Could you check a few things on this model? Use its own coordinates, in mm. Face numbers are marked on the shaded views. Give positions to 0.01 mm unless a question says otherwise; leave off trailing zeros. Order: outer loops, then holes, each group sorted by start corner. A loop starts at its lowest first (then second) coordinate and runs counter-clockwise, first axis right, second up. Notation, with made-up numbers: (69.25, -17) - (87.25, -17) arc R19 cw to (87.25, 8) - close; hole circle Ø4 at (13.25, 81). An arc over 180 degrees is marked (long way). One line per question, with ' | ' between items. Start each with the question number.
1. Imagine slicing it at D-D (x = 62). Please give me the cut outline in (y, z).
2. Imagine slicing it at C-C (z = -45.9). Please give me the cut outline in (x, y), and give its area (3 significant figures).
3. If we mould it in two halves opening along Z, with no side actions, what happens to the marked faces 1 and 2? For each: released by +Z, released by -Z, zero draft, split by the parting line, or undercut.
4. Imagine slicing it at A-A (z = -17.94). Please give me the cut outline in (x, y).
5. Imagine slicing it at B-B (y = 2.95). Give the number of separate pieces and of enclosed holes in the cut face, and give its area (3 significant figures).
6. I need wall thicknesses on probe 1 along Z at (x, y) = (1, 3.65); probe 2 along Y at (x, z) = (63.5, -30); probe 3 along X at (y, z) = (1.6, -8.5). Which ranges of each line are inside material? Lowest first, please. Write a range as from..to.
7. For P1, Ø3, axis at y = 3, z = -45, coming from the +X side; P2, Ø2, axis at x = 54.12, z = -50.9, coming from the -Y side; P3, Ø2, axis at x = 42.5, y = 4.5, coming from the +Z side; P4, Ø1, axis at x = 54.5, z = -51, coming from the +Y side, each with a flat end and sliding along its axis, tell me the tip position at first contact or that it passes through.
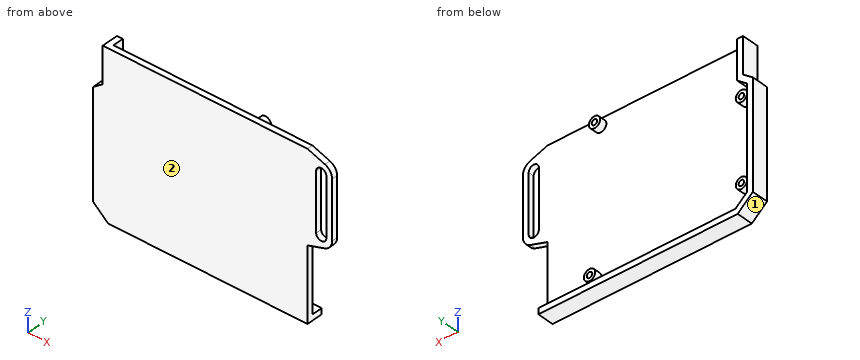
```python
from build123d import *

# Parameters (mm, degrees)
SALIENTE_EXTRUIR2_DEPTH = 2
SALIENTE_EXTRUIR3_DEPTH = 3.7
CROQUIS3_R              = 1.95
CROQUIS3_R_2            = 0.95
SALIENTE_EXTRUIR4_DEPTH = 2.5


with BuildPart() as part:
    # Croquis1 → Saliente-Extruir2 (new body)
    with BuildSketch(Plane(origin=(0, 0, 0), x_dir=(1, 0, 0), z_dir=(0, 1, 0))):
        with BuildLine():
            Line((70.799071053, 31.092568315), (70.799071053, 56.4))
            Line((70.799071053, 56.4), (1.865918726, 56.4))
            Line((1.865918726, 56.4), (-3.400928947, 51.75405083))
            Line((-3.400928947, 51.75405083), (-3.400928947, 14.921940047))
            Line((-3.400928947, 14.921940047), (0, 12.421940047))
            Line((0, 12.421940047), (0, 0))
            Line((0, 0), (70.799071053, 0))
            Line((70.799071053, 0), (76.842269578, 2.170786153))
            ThreePointArc((76.842269578, 2.170786153), (78.641822821, 3.542629227), (79.324535526, 5.7))
            Line((79.324535526, 5.7), (79.324535526, 25.7))
            ThreePointArc((79.324535526, 25.7), (78.590944159, 27.927953986), (76.677186746, 29.284223805))
            Line((76.677186746, 29.284223805), (70.799071053, 31.092568315))
        make_face()
        with BuildLine():
            Line((77.324535526, 25.7), (77.324535526, 5.7))
            ThreePointArc((77.324535526, 5.7), (75.574535526, 3.95), (73.824535526, 5.7))
            Line((73.824535526, 5.7), (73.824535526, 25.7))
            ThreePointArc((73.824535526, 25.7), (75.574535526, 27.45), (77.324535526, 25.7))
        make_face(mode=Mode.SUBTRACT)
    extrude(amount=SALIENTE_EXTRUIR2_DEPTH)

    # Croquis2 → Saliente-Extruir3 (add)
    with BuildSketch(Plane(origin=(0, 2, 0), x_dir=(1, 0, 0), z_dir=(0, 1, 0))):
        Polygon((70.799071053, 54.4), (2.621972909, 54.4), (-1.400928947, 50.851350277), (-1.400928947, 15.933980016), (2, 13.433980016), (2, 0), (0, 0), (0, 12.421940047), (-3.400928947, 14.921940047), (-3.400928947, 51.75405083), (1.865918726, 56.4), (70.799071053, 56.4), align=None)
    extrude(amount=SALIENTE_EXTRUIR3_DEPTH)

    # Croquis3 → Saliente-Extruir4 (add)
    # profile 1 of 4: a face of its own
    with BuildSketch(Plane(origin=(0, 2, 0), x_dir=(1, 0, 0), z_dir=(0, 1, 0))):
        with Locations(Location((1.599071053, 45.9, 0), (0, 0, 270))):
            Circle(CROQUIS3_R)
        with Locations(Location((1.599071053, 45.9, 0), (0, 0, 270))):
            Circle(CROQUIS3_R_2, mode=Mode.SUBTRACT)
    # profile 2 of 4: a face of its own
    with BuildSketch(Plane(origin=(0, 2, 0), x_dir=(1, 0, 0), z_dir=(0, 1, 0))):
        with Locations(Location((1.599071053, 17.94, 0), (0, 0, 270))):
            Circle(CROQUIS3_R)
        with Locations(Location((1.599071053, 17.94, 0), (0, 0, 270))):
            Circle(CROQUIS3_R_2, mode=Mode.SUBTRACT)
    # profile 3 of 4: a face of its own
    with BuildSketch(Plane(origin=(0, 2, 0), x_dir=(1, 0, 0), z_dir=(0, 1, 0))):
        with Locations(Location((52.409071053, 2.505, 0), (0, 0, 270))):
            Circle(CROQUIS3_R)
        with Locations(Location((52.409071053, 2.505, 0), (0, 0, 270))):
            Circle(CROQUIS3_R_2, mode=Mode.SUBTRACT)
    # profile 4 of 4: a face of its own
    with BuildSketch(Plane(origin=(0, 2, 0), x_dir=(1, 0, 0), z_dir=(0, 1, 0))):
        with Locations(Location((54.119071053, 50.9, 0), (0, 0, 270))):
            Circle(CROQUIS3_R)
        with Locations(Location((54.119071053, 50.9, 0), (0, 0, 270))):
            Circle(CROQUIS3_R_2, mode=Mode.SUBTRACT)
    extrude(amount=SALIENTE_EXTRUIR4_DEPTH)


solid = part.part
```
Results found:
1) outline: (0, -56.4) - (5.7, -56.4) - (5.7, -54.4) - (2, -54.4) - (2, 0) - (0, 0) - close
2) outline: (-3.4, 0) - (70.8, 0) - (70.8, 2) - (3.55, 2) - (3.55, 4.5) - (2.55, 4.5) - (2.55, 2) - (0.65, 2) - (0.65, 4.5) - (-0.35, 4.5) - (-0.35, 2) - (-1.4, 2) - (-1.4, 5.7) - (-3.4, 5.7) - close | area: 161 mm2
3) face 1: released by -Z | face 2: zero draft
4) outline: (-3.4, 0) - (73.82, 0) - (73.82, 2) - (3.55, 2) - (3.55, 4.5) - (2.55, 4.5) - (2.55, 2) - (0.65, 2) - (0.65, 4.5) - (-0.35, 4.5) - (-0.35, 2) - (-1.4, 2) - (-1.4, 5.7) - (-3.4, 5.7) - close; (77.32, 0) - (79.32, 0) - (79.32, 2) - (77.32, 2) - close
5) separate pieces: 5 | enclosed holes: 4 | area: 292 mm2
6) probe 1: z = -55.64..-52.97, -47.76..-46.64, -45.16..-44.04, -19.8..-18.68, -17.2..-16.08, -14.17..0 | probe 2: y = 0..2 | probe 3: x = 0..73.82, 77.32..79.32
7) P1: stops at x = 70.8 | P2: stops at y = 0 | P3: stops at z = -54.4 | P4: stops at y = 2
